```python
from build123d import *

# Parameters (mm, degrees)
SKETCH1_R                = 1.5
BOSS_EXTRUDE1_DEPTH      = 1.5
BOSS_EXTRUDE1_DEPTH_BACK = 1.5


with BuildPart() as part:
    # Sketch1 → Boss-Extrude1 (new body, two sides)
    with BuildSketch(Plane(origin=(0, 0, 0), x_dir=(1, 0, 0), z_dir=(0, 1, 0))) as boss_extrude1_sk:
        with BuildLine():
            Line((-14, 35), (-20, 7.5))
            ThreePointArc((-20, 7.5), (-27.5, 0), (-20, -7.5))
            Line((-20, -7.5), (-14, -33))
            Line((-14, -33), (14, -33))
            Line((14, -33), (20, -7.5))
            ThreePointArc((20, -7.5), (27.5, 0), (20, 7.5))
            Line((20, 7.5), (14, 35))
            Line((14, 35), (-14, 35))
        make_face()
        with Locations((0, -20)):
            Circle(SKETCH1_R, mode=Mode.SUBTRACT)
        with Locations((0, 20)):
            Circle(SKETCH1_R, mode=Mode.SUBTRACT)
        with Locations((-7, -28)):
            Circle(SKETCH1_R, mode=Mode.SUBTRACT)
        with Locations((-7, 30)):
            Circle(SKETCH1_R, mode=Mode.SUBTRACT)
        with Locations((-20, 0)):
            Circle(SKETCH1_R, mode=Mode.SUBTRACT)
        with Locations((7, 30)):
            Circle(SKETCH1_R, mode=Mode.SUBTRACT)
        with Locations((7, -28)):
            Circle(SKETCH1_R, mode=Mode.SUBTRACT)
        with Locations((20, 0)):
            Circle(SKETCH1_R, mode=Mode.SUBTRACT)
    extrude(amount=BOSS_EXTRUDE1_DEPTH)
    extrude(boss_extrude1_sk.sketch, amount=-BOSS_EXTRUDE1_DEPTH_BACK)


solid = part.part
```
Geometry check sheet. Reference: the model listing, model coordinates, mm. Coordinates: 2 decimals unless noted, no trailing zeros. Loops run counter-clockwise (first coordinate to the right, second up) from the corner with the lowest first, then second, coordinate; pieces in that order, holes last. Notation, with made-up numbers: (55.5, 62) -> (71.5, 62) arc R20 ccw to (71.5, 70) -> close; hole circle Ø1 at (73.5, 27.5). An arc over 180 degrees is marked (long way). Put each result on its own line as item: value.
1) Gauge pin test, flat ends, axial feed: pin 1 Ø5 at (x, z) = (0, -20) entering from -Y; pin 2 Ø1.8 at (x, z) = (-20, 0) entering from -Y. Record the tip position at first contact, or that the pin passes through.
Result set:
pin 1: stops at y = -1.5
pin 2: passes through
2) Cross-section at D-D on z = 15.5. Record the boundary of the cut face in (x, y).
Result set:
outline: (-18.12, -1.5) -> (18.12, -1.5) -> (18.12, 1.5) -> (-18.12, 1.5) -> close
3) Release check for a two-part mould opening along X. For faces 1 (the flat face through (-16.96, 0.02, -21.44)), 2 (the flat face through (0, 0, -35)), 3 (the cylindrical face through (-8.11, -0.02, -31.01)) record: released by +X, released by -X, zero draft, split by the parting line, or undercut.
Result set:
face 1: released by -X
face 2: zero draft
face 3: undercut
4) Cross-section at A-A on z = 0. Record the boundary of the cut face in (x, y).
Result set:
outline: (-27.5, -1.5) -> (-21.5, -1.5) -> (-21.5, 1.5) -> (-27.5, 1.5) -> close; (-18.5, -1.5) -> (18.5, -1.5) -> (18.5, 1.5) -> (-18.5, 1.5) -> close; (21.5, -1.5) -> (27.5, -1.5) -> (27.5, 1.5) -> (21.5, 1.5) -> close
5) Cross-section at B-B on y = 0.8. Count the separate pieces of the cut face and the enclosed holes in it, plus the area to 3 significant figures.
Result set:
separate pieces: 1
enclosed holes: 8
area: 2,520 mm^2
6) Cross-section at C-C on x = -7. Record the boundary of the cut face in (y, z), plus the area to 3 significant figures.
Result set:
outline: (-1.5, -35) -> (1.5, -35) -> (1.5, -31.5) -> (-1.5, -31.5) -> close; (-1.5, -28.5) -> (1.5, -28.5) -> (1.5, 26.5) -> (-1.5, 26.5) -> close; (-1.5, 29.5) -> (1.5, 29.5) -> (1.5, 33) -> (-1.5, 33) -> close
area: 186 mm^2
7) Thickness scan on line 1 (Z direction, x = 0, y = -0.1); line 2 (Z direction, x = 7, y = 0.2); line 3 (X direction, y = -0.6, z = 0). Record the ranges inside material, lowest first.
Result set:
line 1: z = -35 to -21.5, -18.5 to 18.5, 21.5 to 33
line 2: z = -35 to -31.5, -28.5 to 26.5, 29.5 to 33
line 3: x = -27.5 to -21.5, -18.5 to 18.5, 21.5 to 27.5
